Verification items for the finished model (mm, model axes). A direction names the side the tool comes from. Coordinates: 2 decimals unless noted, no trailing zeros. Loops run counter-clockwise (first coordinate to the right, second up) from the corner with the lowest first, then second, coordinate; pieces in that order, holes last. Notation, with made-up numbers: (41, -2) - (79, -2) arc R7 cw to (79, 9) - close; hole circle Ø11 at (43, -13). An arc over 180 degrees is marked (long way). One line per item, written item: value. Start each with the question number.
(1) Draft check along Z on faces 1 (the face through (9.63, 5.65, -2.01)), 2 (the face through (2, 4.3, -3)), 3 (the face through (18, 4, 0)), 4 (the face through (23.46, 2.9, -2.38)). Enter one of: +Z half, -Z half, draft (parallel to the pull), parting line (faces both ways), or undercut.
(2) Section check A-A (y = 6.75). Record the boundary of the cut face in (x, z).
(3) Thickness scan on probe 1 along X at (y, z) = (4.75, -2.5); probe 2 along Z at (x, y) = (9, 4.8); probe 3 along X at (y, z) = (5.25, -2.05). Record the ranges inside material, lowest first. Write a range as [from, to].
(4) Gauge pin test, flat ends, axial feed: P1, Ø1.3, axis at x = 23.4, z = -2.5, coming from the +Y side; P2, Ø3, axis at x = 1.5, z = -2, coming from the +Y side; P3, Ø2, axis at y = 7, z = -3.5, coming from the -X side. Record the tip position at first contact, or that the pin passes through.
(5) Set-up check for faces 5 (the face through (4, 6, -2)), 6 (the face through (24.2, 5.7, -2.5)), 7 (the face through (28.4, 6, -2)): record each of +Z, -Z, +X, -X, +Y, -Y from which the full face is reachable in a straight line by a thin tool's end or side.
```python
from build123d import *

# Parameters (mm, degrees)
SKETCH2_W                       = 36.4
SKETCH2_H                       = 5
BOSS_EXTRUDE1_DEPTH             = 4.3
SKETCH3_W                       = 24.4
SKETCH3_H                       = 5
BOSS_EXTRUDE2_DEPTH             = 4
M2X0_4_TAPPED_HOLE1_D           = 1.6
M2X0_4_TAPPED_HOLE1_DEPTH       = 5
M2X0_4_TAPPED_HOLE1_CSINK_D     = 2.05
M2X0_4_TAPPED_HOLE1_CSINK_ANGLE = 90
M2X0_4_TAPPED_HOLE1_TIP         = 0.480688495


with BuildPart() as part:
    # Sketch2 → Boss-Extrude1 (new body)
    with BuildSketch(Plane(origin=(0, 0, 0), x_dir=(1, 0, 0), z_dir=(0, 1, 0))):
        with Locations((18.2, 2.5)):
            Rectangle(SKETCH2_W, SKETCH2_H)
    extrude(amount=BOSS_EXTRUDE1_DEPTH)

    # Sketch3 → Boss-Extrude2 (add)
    with BuildSketch(Plane(origin=(0, 4.3, 0), x_dir=(1, 0, 0), z_dir=(0, 1, 0))):
        with Locations((16.2, 2.5)):
            Rectangle(SKETCH3_W, SKETCH3_H)
    extrude(amount=BOSS_EXTRUDE2_DEPTH)

    # M2x0.4 Tapped Hole1
    with Locations(Plane(origin=(0, 8.3, 0), x_dir=(1, 0, 0), z_dir=(0, 1, 0))):
        with Locations((9, 2.5), (23.4, 2.5)):
            CounterSinkHole(M2X0_4_TAPPED_HOLE1_D / 2, M2X0_4_TAPPED_HOLE1_CSINK_D / 2, depth=M2X0_4_TAPPED_HOLE1_DEPTH, counter_sink_angle=M2X0_4_TAPPED_HOLE1_CSINK_ANGLE)
            with Locations((0, 0, -(M2X0_4_TAPPED_HOLE1_DEPTH + M2X0_4_TAPPED_HOLE1_TIP / 2))):  # 118° drill point
                Cone(0, M2X0_4_TAPPED_HOLE1_D / 2, M2X0_4_TAPPED_HOLE1_TIP, mode=Mode.SUBTRACT)


solid = part.part
```
Responses:
1. face 1: undercut
1. face 2: draft
1. face 3: +Z half
1. face 4: undercut
2. outline: (4, -5) - (28.4, -5) - (28.4, 0) - (4, 0) - close; hole circle Ø1.6 at (9, -2.5); hole circle Ø1.6 at (23.4, -2.5)
3. probe 1: x = [4, 8.2], [9.8, 22.6], [24.2, 28.4]
3. probe 2: z = [-5, -3.3], [-1.7, 0]
3. probe 3: x = [4, 8.34], [9.66, 22.74], [24.06, 28.4]
4. P1: stops at y = 3.21
4. P2: stops at y = 4.3
4. P3: stops at x = 4
5. face 5: +Z, -Z, -X, +Y
5. face 6: +Y
5. face 7: +Z, -Z, +X, +Y
